from build123d import *

# Parameters (mm, degrees)
SKETCH1_W           = 48
SKETCH1_H           = 100
BOSS_EXTRUDE1_DEPTH = 5
SKETCH2_W           = 20
SKETCH2_H           = 5
BOSS_EXTRUDE2_DEPTH = 5
SKETCH3_R           = 6
BOSS_EXTRUDE3_DEPTH = 5
SKETCH4_R           = 2.5
CUT_EXTRUDE1_DEPTH  = 5
SKETCH5_W           = 53.859094163
SKETCH5_H           = 28.820783856
CUT_EXTRUDE2_DEPTH  = 10


with BuildPart() as part:
    # Sketch1 → Boss-Extrude1 (new body)
    with BuildSketch(Plane.XY):
        Rectangle(SKETCH1_W, SKETCH1_H)
    extrude(amount=BOSS_EXTRUDE1_DEPTH)

    # Sketch2 → Boss-Extrude2 (add)
    with BuildSketch(Plane(origin=(0, 50, 0), x_dir=(1, 0, 0), z_dir=(0, 1, 0))):
        with Locations((0, -2.5)):
            Rectangle(SKETCH2_W, SKETCH2_H)
    boss_extrude2 = extrude(amount=BOSS_EXTRUDE2_DEPTH)

    # Mirror1: Boss-Extrude2 across plane
    add(boss_extrude2.mirror(Plane.ZX))

    # Sketch3 → Boss-Extrude3 (add)
    with BuildSketch(Plane.XY.offset(5)):
        with Locations((0, 52.5)):
            Circle(SKETCH3_R)
    boss_extrude3 = extrude(amount=-BOSS_EXTRUDE3_DEPTH)

    # Sketch4 → Cut-Extrude1 (cut)
    with BuildSketch(Plane.XY.offset(5)):
        with Locations((0, 52.5)):
            Circle(SKETCH4_R)
    cut_extrude1 = extrude(amount=-CUT_EXTRUDE1_DEPTH, mode=Mode.SUBTRACT)

    # Mirror2: Boss-Extrude3, Cut-Extrude1 across plane
    add(boss_extrude3.mirror(Plane.ZX))
    add(cut_extrude1.mirror(Plane.ZX), mode=Mode.SUBTRACT)

    # Sketch5 → Cut-Extrude2 (cut)
    with BuildSketch(Plane.XY.offset(5)):
        with Locations((2.929547082, -44.410391928)):
            Rectangle(SKETCH5_W, SKETCH5_H)
    extrude(amount=-CUT_EXTRUDE2_DEPTH, mode=Mode.SUBTRACT)


solid = part.part
Geometry check sheet. Reference: the model listing, model coordinates, mm. A direction names the side the tool comes from. Give positions to 0.01 mm unless a question says otherwise; leave off trailing zeros. Order: outer loops, then holes, each group sorted by start corner. A loop starts at its lowest first (then second) coordinate and runs counter-clockwise, first axis right, second up. Notation, with made-up numbers: M -39.5,-14 L -30.5,-14 A27 ccw -30.5,14 Z; hole C 50.25,59 d6. An arc over 180 degrees is marked long. Use a Markdown table: item, result.
Item 1: Section check B-B (y = 52.5). Record the cut outline in (x, z), and give its area (3 significant figures).
Answers follow:
| item | result |
|---|---|
| outline | M -10,0 L -2.5,0 L -2.5,5 L -10,5 Z; M 2.5,0 L 10,0 L 10,5 L 2.5,5 Z |
| area | 75.0 mm2 |
Item 2: Section check A-A (z = 2.3). Record the cut outline in (x, y).
Answers follow:
| item | result |
|---|---|
| outline | M -24,-30 L 24,-30 L 24,50 L 10,50 L 10,55 L 5.45,55 A6 ccw -5.45,55 L -10,55 L -10,50 L -24,50 Z; hole C 0,52.5 d5 |
Item 3: Section check C-C (x = -1). Record the cut outline in (y, z).
Answers follow:
| item | result |
|---|---|
| outline | M -30,0 L 50.21,0 L 50.21,5 L -30,5 Z; M 54.79,0 L 58.42,0 L 58.42,5 L 54.79,5 Z |
Item 4: Section check D-D (x = -6.5). Record the cut outline in (y, z), and give its area (3 significant figures).
Answers follow:
| item | result |
|---|---|
| outline | M -30,0 L 55,0 L 55,5 L -30,5 Z |
| area | 425 mm2 |
Item 5: Tool access check on faces 1 (the cylindrical face through (-0.54, 50.06, 2.54)), 2 (the flat face through (8, 55, 2)), 3 (the flat face through (-10, 52, 3)). Record the directions out of +Z, -Z, +X, -X, +Y, -Y that give a thin tool (end or side, any length) a straight path to the whole face; none if there is none.
Answers follow:
| item | result |
|---|---|
| face 1 | +Z, -Z |
| face 2 | +Z, -Z, +X, +Y |
| face 3 | +Z, -Z, -X, +Y |
Item 6: Depth check by flat-ended pin: P1, Ø1, axis at x = -7, y = 38, coming from the -Z side; P2, Ø2.5, axis at x = -18.5, z = 2, coming from the +Y side. Enter the tip coordinate at first touch or a pass-through.
Answers follow:
| item | result |
|---|---|
| P1 | stops at z = 0 |
| P2 | stops at y = 50 |
Item 7: Material ranges on line 1 along Y through (x, z) = (0, 3.6); line 2 along Y through (x, z) = (-21, 1.55); line 3 along Y through (x, z) = (-1, 0.85), recorded low to high.
Answers follow:
| item | result |
|---|---|
| line 1 | y = -30 to 50, 55 to 58.5 |
| line 2 | y = -30 to 50 |
| line 3 | y = -30 to 50.21, 54.79 to 58.42 |
